Autodesk Inventor part; units mm, degrees
ref_plane "ip_st_or_1_XY" through (0, 0, 0) normal (1, 0, 0) x (0, 0, -1)
ref_plane "ip_st_or_1_YZ" through (0, 0, 0) normal (0, 0, -1) x (0, 1, 0)
ref_plane "ip_st_or_1_ZX" through (0, 0, 0) normal (0, 1, 0) x (1, 0, 0)
sketch "Sketch_1" plane through (0, 0, 0) normal (0, 0, 1) x (1, 0, 0)
  line L0 (4, 0) -> (0, 0)
  line L1 (0, 5.45) -> (0.2656, 5.45)
  line L2 (0.2656, 5.45) -> (0.2656, 5.095)
  line L3 (0.2656, 5.095) -> (1.3247, 5.095)
  arc A0 (2.6753, 5.095) -> (1.3247, 5.095) centre (2, 4.5) ccw
  line L4 (2.6753, 5.095) -> (3.7344, 5.095)
  line L5 (3.7344, 5.095) -> (3.7344, 5.45)
  line L6 (3.7344, 5.45) -> (4, 5.45)
  line L7 (4, 5.45) -> (4, 5.85)
  arc A1 (4, 5.85) -> (3.85, 6) centre (3.85, 5.85) ccw
  line L8 (3.85, 6) -> (0.15, 6)
  arc A2 (0.15, 6) -> (0, 5.85) centre (0.15, 5.85) ccw
  line L9 (0, 5.85) -> (0, 5.45)
revolve "Revolution1" add sketch "Sketch_1" angle 360 about axis through (4, 0, 0) along (1, 0, 0)
ref_plane "ip_st_or_1_XY" through (0, 0, 0) normal (1, 0, 0) x (0, 0, -1)
ref_plane "ip_st_or_1_YZ" through (0, 0, 0) normal (0, 0, -1) x (0, 1, 0)
ref_plane "ip_st_or_1_ZX" through (0, 0, 0) normal (0, 1, 0) x (1, 0, 0)
ref_plane "ip_st_or_2_XY" through (3.7344, 0, 0) normal (-1, 0, 0) x (0, 0, -1)
ref_plane "ip_st_or_2_YZ" through (3.7344, 0, 0) normal (0, 0, -1) x (0, -1, 0)
ref_plane "ip_st_or_2_ZX" through (3.7344, 0, 0) normal (0, -1, 0) x (-1, 0, 0)
properties part number "MR126ZZ Outer Ring"
Input: part model. Units: mm. Frame: model coordinates. Round coordinates to 2 decimals unless told otherwise and drop trailing zeros. Write each loop counter-clockwise with the first axis right and the second up, starting at its lowest first coordinate (ties: lowest second). Pieces come first, ordered by that corner, then holes.
1) Cut plane A-A (z = 0). Return the cut outline in (x, y) (3 decimals).
2) Draft query along Y for faces 1 (the cylindrical face through (2, -6, 0)), 2 (the flat face through (4, 4, -4)), 3 (the cylindrical face through (0.803, -1.104, -4.974)). Return one class per face: pulls with the +Y half, pulls with the -Y half, needs draft (parallel to the pull), parting line crosses it, or undercut.
3) Cut plane D-D (x = 1.95). Return the cut outline in (y, z), then the cut area to 3 significant figures.
4) Cut plane C-C (x = 0.5). Return the cut outline in (y, z) (3 decimals), then the cut area to 3 significant figures.
5) Contact query for a flat-ended pin moving along its axis: P1, Ø6, axis at y = 0, z = 0, coming from the -X side. Output: stop coordinate, or through.
6) Ray query, L1, parallel to Z at x = 0.95, y = 0 (3 decimals); L2, parallel to Z at x = 3.85, y = 0; L3, parallel to Y at x = 0.7, z = -2.75. Return the intervals inside material, ascending.
Geometry says:
1. outline: (0, -5.85) arc R0.15 ccw to (0.15, -6) - (3.85, -6) arc R0.15 ccw to (4, -5.85) - (4, -5.45) - (3.734, -5.45) - (3.734, -5.095) - (2.675, -5.095) arc R0.9 cw to (1.325, -5.095) - (0.266, -5.095) - (0.266, -5.45) - (0, -5.45) - close; (0, 5.45) - (0.266, 5.45) - (0.266, 5.095) - (1.325, 5.095) arc R0.9 cw to (2.675, 5.095) - (3.734, 5.095) - (3.734, 5.45) - (4, 5.45) - (4, 5.85) arc R0.15 ccw to (3.85, 6) - (0.15, 6) arc R0.15 ccw to (0, 5.85) - close
2. face 1: parting line crosses it
2. face 2: needs draft
2. face 3: undercut
3. outline: circle Ø12 at (0, 0); hole circle Ø10.8 at (0, 0)
3. area: 21.5 mm2
4. outline: circle Ø12 at (0, 0); hole circle Ø10.19 at (0, 0)
4. area: 31.5 mm2
5. P1: passes through
6. L1: z = -6 to -5.095, 5.095 to 6
6. L2: z = -6 to -5.45, 5.45 to 6
6. L3: y = -5.33 to -4.29, 4.29 to 5.33
